Can you work these out from the model? Positions are in its coordinate system, mm. A direction names the side the tool comes from. Coordinates: 2 decimals unless noted, no trailing zeros. Order: outer loops, then holes, each group sorted by start corner. A loop starts at its lowest first (then second) coordinate and runs counter-clockwise, first axis right, second up. Notation, with made-up numbers: M 50,60 L 74,60 A28 ccw 74,79 Z; hole C -1,9.25 d9. An arc over 180 degrees is marked long. Answer as a JSON object with one key per item and string values.
from build123d import *

# Parameters (mm, degrees)
F1_DEPTH = 12.7
F2_R     = 3.175
F3_DEPTH = 25.4


with BuildPart() as f1:
    # F0 (on Front) → F1 (new body)
    with BuildSketch(Plane.XZ):
        with BuildLine():
            Line((-20.7645, -33.147), (-20.7645, -1.625153))
            ThreePointArc((-20.7645, -1.625153), (0, 20.828), (20.7645, -1.625153))
            Line((20.7645, -1.625153), (20.7645, -33.147))
            Line((20.7645, -33.147), (14.4145, -33.147))
            Line((14.4145, -33.147), (14.4145, -39.497))
            Line((14.4145, -39.497), (27.1145, -39.497))
            Line((27.1145, -39.497), (27.1145, -1.625153))
            ThreePointArc((27.1145, -1.625153), (24.080006, 12.833079), (13.930541, 23.567929))
            ThreePointArc((13.930541, 23.567929), (8.88597, 29.201016), (7.9375, 36.703))
            Line((7.9375, 36.703), (0, 36.703))
            Line((0, 36.703), (-7.9375, 36.703))
            ThreePointArc((-7.9375, 36.703), (-8.88597, 29.201016), (-13.930541, 23.567929))
            ThreePointArc((-13.930541, 23.567929), (-24.080006, 12.833079), (-27.1145, -1.625153))
            Line((-27.1145, -1.625153), (-27.1145, -39.497))
            Line((-27.1145, -39.497), (-14.4145, -39.497))
            Line((-14.4145, -39.497), (-14.4145, -33.147))
            Line((-14.4145, -33.147), (-20.7645, -33.147))
        make_face()
    extrude(amount=F1_DEPTH)

    # F2 (on face) → F3 (cut)
    with BuildSketch(Plane.XY.offset(36.703)):
        with Locations((0, -6.35)):
            Circle(F2_R)
    extrude(amount=-F3_DEPTH, mode=Mode.SUBTRACT)


solid = f1.part
Item 1: Please list where these lines run through material, in increasing order: line 1 (X direction, y = -1.5, z = -7); line 2 (Y direction, x = 0, z = 29) (3 decimals); line 3 (X direction, y = -6.75, z = -0.5).
Answers follow:
{"line 1": "x = -27.11 to -20.76, 20.76 to 27.11", "line 2": "y = -12.7 to -9.525, -3.175 to 0", "line 3": "x = -27.17 to -20.82, 20.82 to 27.17"}
Item 2: I want a section at B-B, the plane z = -22.5. Write out the boundary of the cut face in (x, y), plus the area to 3 significant figures.
Answers follow:
{"outline": "M -27.11,-12.7 L -20.76,-12.7 L -20.76,0 L -27.11,0 Z; M 20.76,-12.7 L 27.11,-12.7 L 27.11,0 L 20.76,0 Z", "area": "161 mm^2"}
Item 3: If we mould it in two halves opening along Y, with no side actions, what happens to faces 1 (the flat face through (-20.764, -6, -18)), 2 (the cylindrical face through (-0.69, -9.45, 28.76)), 3 (the flat face through (20, -12.7, 7))? For each: pulls with the +Y half, pulls with the -Y half, needs draft (parallel to the pull), parting line crosses it, or undercut.
Answers follow:
{"face 1": "needs draft", "face 2": "undercut", "face 3": "pulls with the -Y half"}
Item 4: I want a section at A-A, the plane y = -6.35. Write out the boundary of the cut face in (x, z) (1 decimal).
Answers follow:
{"outline": "M -27.1,-39.5 L -14.4,-39.5 L -14.4,-33.1 L -20.8,-33.1 L -20.8,-1.6 A20.8 cw -3.2,20.6 L -3.2,36.7 L -7.9,36.7 A12.7 cw -13.9,23.6 A27.2 ccw -27.1,-1.6 Z; M 3.2,20.6 A20.8 cw 20.8,-1.6 L 20.8,-33.1 L 14.4,-33.1 L 14.4,-39.5 L 27.1,-39.5 L 27.1,-1.6 A27.2 ccw 13.9,23.6 A12.7 cw 7.9,36.7 L 3.2,36.7 Z"}
Item 5: Which directions (+Z, -Z, +X, -X, +Y, -Y) give clear straight access to the entire face, cutting with the end or side of a thin tool? Please do faces 4 (the flat face through (27.114, -6, -21)), 5 (the flat face through (14.414, -6, -36)), 6 (the flat face through (20.764, -6, -17)).
Answers follow:
{"face 4": "-Z, +X, +Y, -Y", "face 5": "-Z, +Y, -Y", "face 6": "+Y, -Y"}
Item 6: I want a section at C-C, the plane x = 0. Write out the boundary of the cut face in (y, z) (3 decimals), plus the area to 3 significant figures.
Answers follow:
{"outline": "M -12.7,20.828 L -9.525,20.828 L -9.525,36.703 L -12.7,36.703 Z; M -3.175,20.828 L 0,20.828 L 0,36.703 L -3.175,36.703 Z", "area": "101 mm^2"}
Item 7: I want a section at D-D, the plane y = -10.5. Write out the boundary of the cut face in (x, z), plus the area to 3 significant figures.
Answers follow:
{"outline": "M -27.11,-39.5 L -14.41,-39.5 L -14.41,-33.15 L -20.76,-33.15 L -20.76,-1.63 A20.83 cw long 20.76,-1.63 L 20.76,-33.15 L 14.41,-33.15 L 14.41,-39.5 L 27.11,-39.5 L 27.11,-1.63 A27.18 ccw 13.93,23.57 A12.7 cw 7.94,36.7 L -7.94,36.7 A12.7 cw -13.93,23.57 A27.18 ccw -27.11,-1.63 Z", "area": "1,240 mm^2"}
Item 8: I'm going to push flat-ended pins straight in: pin 1 (1 mm diameter, centred on x = -10, z = 24.5, fed in from +Y); pin 2 (6.5 mm diameter, centred on y = -4, z = -10, fed in from +X); pin 3 (1.9 mm diameter, centred on x = -17.5, y = -8.5, fed in from +Z); pin 4 (3 mm diameter, centred on x = 17, y = -8, fed in from +Z). Where does each tip first touch, or does it pass through?
Answers follow:
{"pin 1": "stops at y = 0", "pin 2": "stops at x = 27.11", "pin 3": "stops at z = 21.79", "pin 4": "stops at z = 22.56"}
